Verification items for the finished model (mm, model axes). Give positions to 0.01 mm unless a question says otherwise; leave off trailing zeros. Order: outer loops, then holes, each group sorted by start corner. A loop starts at its lowest first (then second) coordinate and runs counter-clockwise, first axis right, second up. Notation, with made-up numbers: (3.25, -30) - (24.25, -30) arc R10 cw to (24.25, -20) - close; hole circle Ø11 at (20, 23). An arc over 180 degrees is marked (long way). Answer as a JSON object with one key per item and string values.
```python
from build123d import *

# Parameters (mm, degrees)
EXTRUDE_START             = -17.5
SKETCH_1_R                = 3
EXTRUDE_231_DEPTH         = 35
SKETCH_2_W                = 16
SKETCH_2_H                = 1.5
EXTRUDE_300_DEPTH         = 35
D3P2_START                = -20
SKETCH_3_R                = 1.6
D3P2_DEPTH                = 40
CUT_EXTRUDE_M3_DEPTH      = 100
CUT_EXTRUDE_M3_DEPTH_BACK = 100
SKETCH_4_R                = 1.6
CUT_EXTRUDE_3_DEPTH       = 100
CUT_EXTRUDE_3_DEPTH_BACK  = 100
SKETCH_5_R                = 1.6


with BuildPart() as part:
    # 草图1 → Extrude 231 (new body)
    with BuildSketch(Plane.XY.offset(EXTRUDE_START)):
        Circle(SKETCH_1_R)
    extrude(amount=EXTRUDE_231_DEPTH)

    # 草图2 → Extrude 300 (add)
    with BuildSketch(Plane.XY.offset(EXTRUDE_START)):
        with Locations((6, -2.25)):
            Rectangle(SKETCH_2_W, SKETCH_2_H)
    extrude(amount=EXTRUDE_300_DEPTH)

    # 草图3 → D3p2活动转轴孔 (cut)
    with BuildSketch(Plane.XY.offset(D3P2_START)):
        Circle(SKETCH_3_R)
    extrude(amount=D3P2_DEPTH, mode=Mode.SUBTRACT)

    # 草图4 → 吊板M3安装孔 (cut, two sides: drawn at the far end of the back side and taken through both)
    with BuildSketch(Plane(origin=(0, 0, 0), x_dir=(1, 0, 0), z_dir=(0, 1, 0)).offset(-CUT_EXTRUDE_M3_DEPTH_BACK)):
        with Locations(Location((8, 12, 0), (0, 0, 270))):
            Circle(SKETCH_4_R)
    extrude(amount=CUT_EXTRUDE_M3_DEPTH + CUT_EXTRUDE_M3_DEPTH_BACK, mode=Mode.SUBTRACT)

    # 草图5 → 切除-拉伸3 (cut, two sides: drawn at the far end of the back side and taken through both)
    with BuildSketch(Plane(origin=(0, 0, 0), x_dir=(1, 0, 0), z_dir=(0, 1, 0)).offset(-CUT_EXTRUDE_3_DEPTH_BACK)):
        with Locations(Location((8, -12, 0), (0, 0, 270))):
            Circle(SKETCH_5_R)
    extrude(amount=CUT_EXTRUDE_3_DEPTH + CUT_EXTRUDE_3_DEPTH_BACK, mode=Mode.SUBTRACT)


solid = part.part
```
(1) Section check A-A (z = -12). Record the cut outline in (x, y).
Computed values:
{"outline": "(-2, -3) - (6.4, -3) - (6.4, -1.5) - (2.6, -1.5) arc R3 ccw (long way) to (-2, -2.24) - close; (9.6, -3) - (14, -3) - (14, -1.5) - (9.6, -1.5) - close; hole circle Ø3.2 at (0, 0)"}
(2) Gauge pin test, flat ends, axial feed: pin 1 Ø3.5 at (x, z) = (8, -12) entering from +Y; pin 2 Ø10 at (x, z) = (6, 4.5) entering from +Y; pin 3 Ø3 at (y, z) = (-2, 1) entering from -X. Record the tip position at first contact, or that the pin passes through.
Computed values:
{"pin 1": "stops at y = -1.5", "pin 2": "stops at y = 2.83", "pin 3": "stops at x = -2.96"}
(3) Release check for a two-part mould opening along Z. For faces 1 (the flat face through (3, -2, -17.5)), 2 (the cylindrical face through (8.07, -2.26, 10.4)), 3 (the flat face through (14, -2, 0)), 4 (the flat face through (3, -2, 17.5)) record: pulls with the +Z half, pulls with the -Z half, needs draft (parallel to the pull), parting line crosses it, or undercut.
Computed values:
{"face 1": "pulls with the -Z half", "face 2": "undercut", "face 3": "needs draft", "face 4": "pulls with the +Z half"}
(4) Section check D-D (x = 8). Record the cut outline in (y, z).
Computed values:
{"outline": "(-3, -17.5) - (-1.5, -17.5) - (-1.5, -13.6) - (-3, -13.6) - close; (-3, -10.4) - (-1.5, -10.4) - (-1.5, 10.4) - (-3, 10.4) - close; (-3, 13.6) - (-1.5, 13.6) - (-1.5, 17.5) - (-3, 17.5) - close"}
(5) Material ranges on line 1 along Z through (x, y) = (8, -1.95); line 2 along X through (y, z) = (-2.3, -12); line 3 along X through (y, z) = (0, 3), recorded low to high. Write a range as [from, to].
Computed values:
{"line 1": "z = [-17.5, -13.6], [-10.4, 10.4], [13.6, 17.5]", "line 2": "x = [-2, 6.4], [9.6, 14]", "line 3": "x = [-3, -1.6], [1.6, 3]"}
(6) Section check B-B (y = 0). Record the cut outline in (x, z).
Computed values:
{"outline": "(-3, -17.5) - (-1.6, -17.5) - (-1.6, 17.5) - (-3, 17.5) - close; (1.6, -17.5) - (3, -17.5) - (3, 17.5) - (1.6, 17.5) - close"}
